Source: CAD feature listing. Evaluate the final solid. Frame: model axes, mm. A direction names the side the tool comes from. Give positions to 0.01 mm unless a question says otherwise; leave off trailing zeros. Order: outer loops, then holes, each group sorted by start corner. A loop starts at its lowest first (then second) coordinate and runs counter-clockwise, first axis right, second up.
Autodesk Inventor part; units mm, degrees
ref_plane "YZ Plane" through (0, 0, 0) normal (1, 0, 0) x (0, 1, 0)
ref_plane "XZ Plane" through (0, 0, 0) normal (0, 1, 0) x (-1, 0, 0)
ref_plane "XY Plane" through (0, 0, 0) normal (0, 0, 1) x (1, 0, 0)
sketch "Sketch1" plane through (0, 0, 0) normal (0, 1, 0) x (-1, 0, 0)
  line L0 (-25, 25) -> (25, 25)
  line L1 (25, 25) -> (25, -25)
  line L2 (25, -25) -> (-25, -25)
  line L3 (-25, -25) -> (-25, 25)
  line L4 (-25, 25) -> (25, -25) construction
  line L5 (25, 25) -> (-25, -25) construction
  circle A0 centre (15, -15) radius 5
  circle A1 centre (-15, -15) radius 5
  circle A2 centre (15, 15) radius 5
  circle A3 centre (-15, 15) radius 5
  circle A4 centre (0, 0) radius 10
  dimension "d0" = 50
  dimension "d1" = 50
  dimension "d2" = 10
  dimension "d3" = 10
  dimension "d6" = 30
  dimension "d9" = 30
  dimension "d12" = 20
extrude "Extrusion1" add sketch "Sketch1" along normal blind 150 contours A4
extrude "Extrusion2" add sketch "Sketch1" against normal blind 10 contours L0 L1 L2 L3 | A4
thread "Thread1"
thread "Thread2"
thread "Thread3"
thread "Thread4"
sketch "Sketch2" plane through (0, 150, 0) normal (0, 1, 0) x (1, 0, 0)
  line L0 (25, 25) -> (-25, 25)
  line L1 (-25, 25) -> (-25, -25)
  line L2 (-25, -25) -> (25, -25)
  line L3 (25, -25) -> (25, 25)
  point P0 (0, 0)
extrude "Extrusion3" add sketch "Sketch2" along normal blind 50
shell "Shell1" thickness 5 removed faces 1 at (-8.3333, 166.6667, 25)
equation "\"d1\" = d0"
equation "\"d3\" = d2"
properties part number "camera_pole"
1) Section query A-A on x = -15. Output: boundary loops of the cut face in (y, z), and give its area (3 significant figures).
Checks:
outline: (-10, -25) - (0, -25) - (0, -20) - (-10, -20) - close; (-10, -10) - (0, -10) - (0, 10) - (-10, 10) - close; (-10, 20) - (0, 20) - (0, 25) - (-10, 25) - close; (150, -25) - (200, -25) - (200, 25) - (195, 25) - (195, -20) - (155, -20) - (155, 25) - (150, 25) - close
area: 1,000 mm2
2) First-contact query: pin 1 Ø10 at (x, z) = (18.5, 16.5) entering from -Y; pin 2 Ø6 at (x, z) = (-15, -15) entering from -Y; pin 3 Ø12 at (x, y) = (2, 183) entering from +Z. Flat tips, straight axial feed; report the tip coordinate or a pass-through.
Checks:
pin 1: stops at y = -10
pin 2: stops at y = 150
pin 3: stops at z = -20
3) Section query C-C on y = 181.5. Output: boundary loops of the cut face in (x, z).
Checks:
outline: (-25, -25) - (25, -25) - (25, 25) - (20, 25) - (20, -20) - (-20, -20) - (-20, 25) - (-25, 25) - close
4) Pull-direction query (Y, two-part tool) for faces 1 (the face through (0, 150, -11)), 2 (the face through (16.08, -4.93, 10.12)), 3 (the face through (0, -10, 0)); classes: +Y half, -Y half, draft (parallel to the pull), parting line (faces both ways), or undercut.
Checks:
face 1: undercut
face 2: draft
face 3: -Y half
5) Section query B-B on z = 15. Output: boundary loops of the cut face in (x, y), and give its area (3 significant figures).
Checks:
outline: (-25, -10) - (-20, -10) - (-20, 0) - (-25, 0) - close; (-25, 150) - (25, 150) - (25, 200) - (-25, 200) - close; (-10, -10) - (10, -10) - (10, 0) - (-10, 0) - close; (20, -10) - (25, -10) - (25, 0) - (20, 0) - close; hole (-20, 155) - (20, 155) - (20, 195) - (-20, 195) - close
area: 1,200 mm2
6) Reachability of faces 4 (the face through (25, 175, 0)), 5 (the face through (0, 197, 25)), 6 (the face through (2.17, 73.95, 9.76)), 7 (the face through (20, 175, 3)), 8 (the face through (16.08, -4.93, -19.88)) from +Z, -Z, +X, -X, +Y, -Y: full face, straight path, thin tool, end or side. Return the list, or none.
Checks:
face 4: +Z, -Z, +X, +Y, -Y
face 5: +Z, +X, -X, +Y, -Y
face 6: none
face 7: +Z
face 8: -Y
7) Ray query, L1, parallel to Y at x = -13, z = 23; L2, parallel to Z at x = 15, y = -2.5; L3, parallel to X at y = 182, z = 2.5. Return the intervals inside material, ascending.
Checks:
L1: y = -10 to 0, 150 to 155, 195 to 200
L2: z = -25 to -20, -10 to 10, 20 to 25
L3: x = -25 to -20, 20 to 25
8) Section query D-D on x = 0. Output: boundary loops of the cut face in (y, z), and give its area (3 significant figures).
Checks:
outline: (-10, -25) - (0, -25) - (0, -10) - (150, -10) - (150, -25) - (200, -25) - (200, 25) - (195, 25) - (195, -20) - (155, -20) - (155, -5) - (-5, -5) - (-5, 5) - (155, 5) - (155, 25) - (150, 25) - (150, 10) - (0, 10) - (0, 25) - (-10, 25) - close
area: 2,600 mm2
